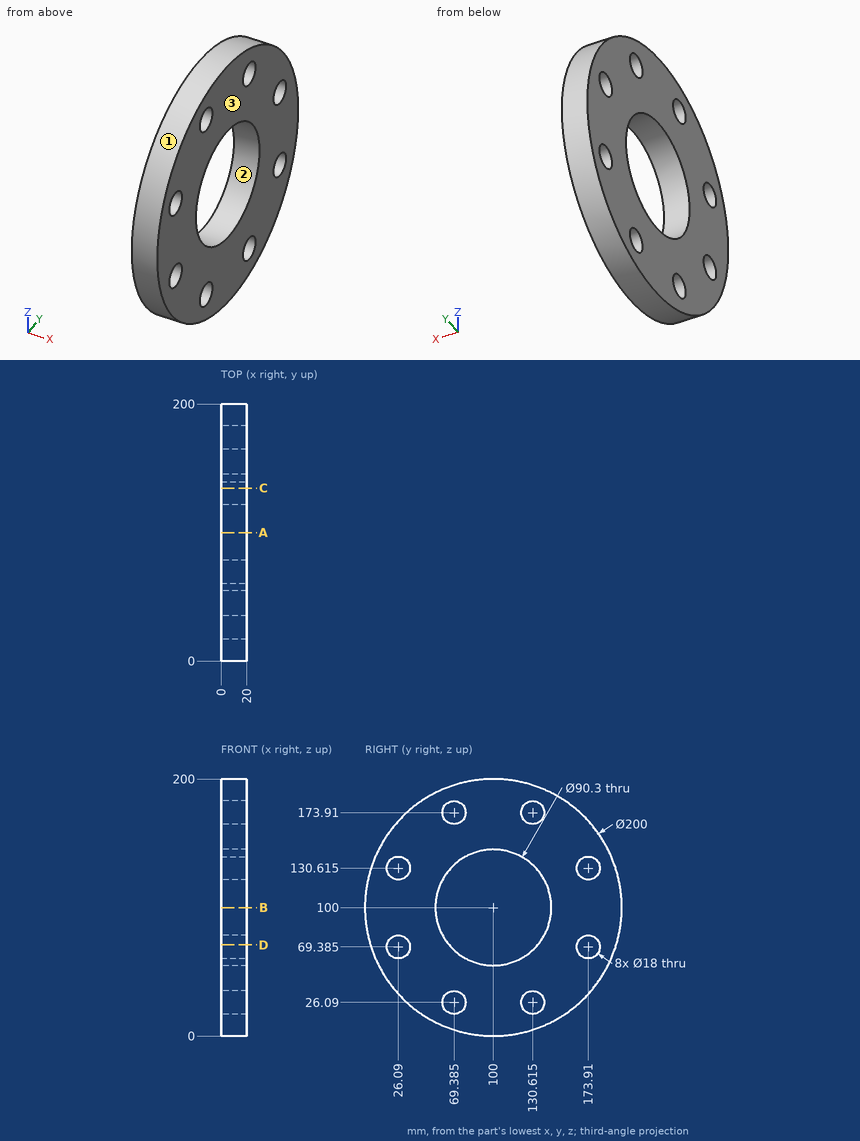
Here's the drawing with two shaded views (mm, measured from the low corner). I have some questions. Coordinates: 2 decimals unless noted, no trailing zeros. Loops run counter-clockwise (first coordinate to the right, second up) from the corner with the lowest first, then second, coordinate; pieces in that order, holes last. Notation, with made-up numbers: M 75.5,-14 L 96.5,-14 A23 cw 96.5,4 Z; hole C 44.25,40 d3. An arc over 180 degrees is marked long. Answer as CSV lines item,"result". Start each with the question number.
1. Thinking about a two-plate mould opening in Y: for the marked faces 1, 2 and 3, which applies, +Y half, -Y half, draft (parallel to the pull), parting line (faces both ways), or undercut?
2. Suppose I cut it at A-A, the plane y = 100. List the corners of the cut face in (x, z) for me.
3. Suppose I cut it at C-C, the plane y = 134.5. List the corners of the cut face in (x, z) for me (1 decimal), plus the area to 3 significant figures.
4. If I drill on probe 1 along Z at (x, y) = (11.25, 67.5); probe 2 along Y at (x, z) = (12.25, 98.5) (1 decimal); probe 3 along Z at (x, y) = (7, 29), over which ranges is the centre line in solid material (lowest first)? Write a range as [from, to].
5. For pin 1 Ø3 at (x, z) = (3.5, 172) entering from -Y; pin 2 Ø6 at (x, z) = (4, 88) entering from +Y; pin 3 Ø12 at (x, y) = (11.5, 175) entering from +Z, each with a flat end and sliding along its axis, tell me the tip position at first contact or that it passes through.
6. Suppose I cut it at D-D, the plane z = 71. List the corners of the cut face in (x, y) for me (1 decimal).
Output:
1,face 1,"parting line"
1,face 2,"undercut"
1,face 3,"draft"
2,outline,"M 0,0 L 20,0 L 20,54.85 L 0,54.85 Z; M 0,145.15 L 20,145.15 L 20,200 L 0,200 Z"
3,outline,"M 0,6.1 L 20,6.1 L 20,18 L 0,18 Z; M 0,34.2 L 20,34.2 L 20,70.9 L 0,70.9 Z; M 0,129.1 L 20,129.1 L 20,165.8 L 0,165.8 Z; M 0,182 L 20,182 L 20,193.9 L 0,193.9 Z"
3,area,"1,940 mm^2"
4,probe 1,"z = [5.43, 17.29], [34.89, 68.66], [131.34, 165.11], [182.71, 194.57]"
4,probe 2,"y = [0, 54.9], [145.1, 200]"
4,probe 3,"z = [29.58, 60.87], [77.9, 122.1], [139.13, 170.42]"
5,pin 1,"stops at y = 29.08"
5,pin 2,"stops at y = 199.59"
5,pin 3,"stops at z = 172.38"
6,outline,"M 0,4.3 L 20,4.3 L 20,17.2 L 0,17.2 Z; M 0,34.9 L 20,34.9 L 20,65.4 L 0,65.4 Z; M 0,134.6 L 20,134.6 L 20,165.1 L 0,165.1 Z; M 0,182.8 L 20,182.8 L 20,195.7 L 0,195.7 Z"
